from build123d import *

# Parameters (mm, degrees)
BOSS_EXTRUDE1_DEPTH = 40
BOSS_EXTRUDE2_DEPTH = 7
BOSS_EXTRUDE3_START = 25
BOSS_EXTRUDE3_DEPTH = 25
BOSS_EXTRUDE4_START = -12
BOSS_EXTRUDE4_DEPTH = 3


with BuildPart() as part:
    # Sketch1 → Boss-Extrude1 (new body)
    with BuildSketch(Plane.XY):
        with BuildLine():
            Line((-2.25, 5.25), (2.25, 5.25))
            ThreePointArc((2.25, 5.25), (4.371320344, 4.371320344), (5.25, 2.25))
            Line((5.25, 2.25), (5.25, -2.25))
            ThreePointArc((5.25, -2.25), (4.371320344, -4.371320344), (2.25, -5.25))
            Line((2.25, -5.25), (-2.25, -5.25))
            ThreePointArc((-2.25, -5.25), (-4.371320344, -4.371320344), (-5.25, -2.25))
            Line((-5.25, -2.25), (-5.25, 2.25))
            ThreePointArc((-5.25, 2.25), (-4.371320344, 4.371320344), (-2.25, 5.25))
        make_face()
    extrude(amount=BOSS_EXTRUDE1_DEPTH)

    # Sketch2 → Boss-Extrude2 (add)
    with BuildSketch(Plane.XY):
        with BuildLine():
            Line((8.999999945, -3.000810302), (8.999999945, 2.999189698))
            ThreePointArc((8.999999945, 2.999189698), (8.121463527, 5.120366794), (6.000405096, 5.999189671))
            Line((6.000405096, 5.999189671), (-5.999594794, 6.000810275))
            ThreePointArc((-5.999594794, 6.000810275), (-8.121177041, 5.122273883), (-8.999999945, 3.000810302))
            Line((-8.999999945, 3.000810302), (-8.999999945, -2.999189698))
            ThreePointArc((-8.999999945, -2.999189698), (-8.121463527, -5.120366794), (-6.000405096, -5.999189671))
            Line((-6.000405096, -5.999189671), (5.999594794, -6.000810275))
            ThreePointArc((5.999594794, -6.000810275), (8.121177041, -5.122273883), (8.999999945, -3.000810302))
        make_face()
    extrude(amount=-BOSS_EXTRUDE2_DEPTH)

    # Sketch3 → Boss-Extrude3 (add)
    with BuildSketch(Plane.XY.offset(BOSS_EXTRUDE3_START)):
        with BuildLine():
            Line((0.000405151, 5.25), (-5.999999945, 5.25))
            ThreePointArc((-5.999999945, 5.25), (-7.590417233, 4.59122759), (-8.249189643, 3.000810302))
            Line((-8.249189643, 3.000810302), (-8.249189643, -2.999189698))
            ThreePointArc((-8.249189643, -2.999189698), (-7.590631979, -4.58939221), (-6.000607381, -5.248379314))
            Line((-6.000607381, -5.248379314), (0.000405151, -5.25))
            Line((0.000405151, -5.25), (0.000405151, -6.000000082))
            Line((0.000405151, -6.000000082), (-6.000405096, -5.999189671))
            ThreePointArc((-6.000405096, -5.999189671), (-8.121463527, -5.120366794), (-8.999999945, -2.999189698))
            Line((-8.999999945, -2.999189698), (-8.999999945, 3.000810302))
            ThreePointArc((-8.999999945, 3.000810302), (-8.121177041, 5.122273883), (-5.999594794, 6.000810275))
            Line((-5.999594794, 6.000810275), (0.000405151, 5.999999973))
            Line((0.000405151, 5.999999973), (0.000405151, 5.25))
        make_face()
    extrude(amount=-BOSS_EXTRUDE3_DEPTH)

    # Sketch5 → Boss-Extrude4 (add)
    with BuildSketch(Plane.XY.offset(40).offset(BOSS_EXTRUDE4_START)):
        with BuildLine():
            Line((0.000405151, -6.000000082), (5.999594794, -6.000810275))
            ThreePointArc((5.999594794, -6.000810275), (8.121177041, -5.122273883), (8.999999945, -3.000810302))
            Line((8.999999945, -3.000810302), (8.999999945, 2.999189698))
            ThreePointArc((8.999999945, 2.999189698), (8.121463527, 5.120366794), (6.000405096, 5.999189671))
            Line((6.000405096, 5.999189671), (0.000405151, 5.999999973))
            Line((0.000405151, 5.999999973), (-5.999594794, 6.000810275))
            ThreePointArc((-5.999594794, 6.000810275), (-8.121177041, 5.122273883), (-8.999999945, 3.000810302))
            Line((-8.999999945, 3.000810302), (-8.999999945, -2.999189698))
            ThreePointArc((-8.999999945, -2.999189698), (-8.121463527, -5.120366794), (-6.000405096, -5.999189671))
            Line((-6.000405096, -5.999189671), (0.000405151, -6.000000082))
        make_face()
    extrude(amount=-BOSS_EXTRUDE4_DEPTH)


solid = part.part
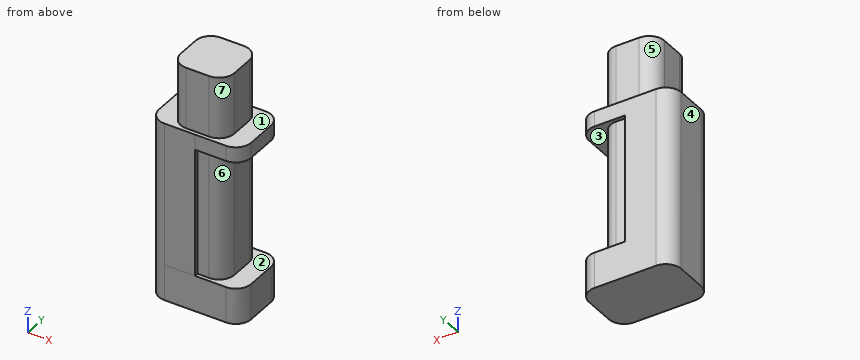
For this review, take the finished solid that the model builds, in its own axes (mm). Face numbers are marked on the shaded views. A direction names the side the tool comes from. Give positions to 0.01 mm unless a question says otherwise; leave off trailing zeros. Order: outer loops, then holes, each group sorted by start corner. A loop starts at its lowest first (then second) coordinate and runs counter-clockwise, first axis right, second up. Notation, with made-up numbers: M 80.25,85.5 L 102.25,85.5 A22 cw 102.25,112.5 Z; hole C 16,74.5 d9. An arc over 180 degrees is marked long. Answer in a Markdown table with one row per item. Add a question column.
(1) Mouldability with a two-part tool opening along Z and no side actions: class the marked faces 1, 2, 3 and 4 as +Z half, -Z half, draft (parallel to the pull), parting line (faces both ways), or undercut.
(2) Consider section D-D on z = -2.5. State the section outline as (x, y) points, and give its area (3 significant figures).
(3) Consider section A-A on z = 6. State the section outline as (x, y) points, and give its area (3 significant figures).
(4) Consider section B-B on y = 0.75. State the section outline as (x, z) points, and give its area (3 significant figures).
(5) Consider section C-C on x = 6.75. State the section outline as (y, z) points.
(6) Wall thickness on probe 1 along Z at (x, y) = (7.5, -0.75); probe 2 along X at (y, z) = (1.25, 23); probe 3 along Y at (x, z) = (2.5, 32.5): over which ranges is each line inside the solid? List them lowest first. Write a range as [from, to].
(7) For the marked faces 5, 6 and 7, list the 3-axis set-ups (+Z, -Z, +X, -X, +Y, -Y) from which the entire face can be reached by the end or side of a thin tool; tool diameter is ignored.
(8) For pin 1 (1.3 mm diameter, centred on y = 1, z = 35, fed in from +X); pin 2 (0.6 mm diameter, centred on y = -6, z = 8, fed in from +X); pin 3 (5 mm diameter, centred on x = 0.5, z = 33.5, fed in from -Y), all flat-tipped, find the tip position at first contact; note any pin that passes through.
Evaluation:
| question | item | result |
|---|---|---|
| 1 | face 1 | +Z half |
| 1 | face 2 | undercut |
| 1 | face 3 | undercut |
| 1 | face 4 | draft |
| 2 | outline | M -9,-3 A3 ccw -6,-6 L 6,-6 A3 ccw 9,-3 L 9,3 A3 ccw 6,6 L -6,6 A3 ccw -9,3 Z |
| 2 | area | 208 mm^2 |
| 3 | outline | M -9,-3 A3 ccw -6,-6 L 0,-6 L 0,-5.25 L 2.25,-5.25 A3 ccw 5.25,-2.25 L 5.25,2.25 A3 ccw 2.25,5.25 L 0,5.25 L 0,6 L -6,6 A3 ccw -9,3 Z; hole M -8.25,-3 A2.25 ccw -6,-5.25 L -2.31,-5.25 A3 cw -5.25,-2.25 L -5.25,2.25 A3 cw -2.25,5.25 L -6,5.25 A2.25 ccw -8.25,3 Z |
| 3 | area | 122 mm^2 |
| 4 | outline | M -9,-7 L 9,-7 L 9,0 L 5.25,0 L 5.25,25 L 9,25 L 9,28 L 5.25,28 L 5.25,40 L -5.25,40 L -5.25,28 L -9,28 Z; hole M -8.25,0 L -5.25,0 L -5.25,25 L -8.25,25 Z |
| 4 | area | 587 mm^2 |
| 5 | outline | M -5.91,-7 L 5.9,-7 L 5.9,0 L -5.91,0 Z; M -5.91,25 L 5.9,25 L 5.9,28 L -5.91,28 Z |
| 6 | probe 1 | z = [-7, 0], [25, 28] |
| 6 | probe 2 | x = [-9, -8.25], [-5.25, 5.25] |
| 6 | probe 3 | y = [-5.24, 5.24] |
| 7 | face 5 | +Z, -X, +Y |
| 7 | face 6 | +X, -Y |
| 7 | face 7 | +Z, +X, -Y |
| 8 | pin 1 | stops at x = 5.25 |
| 8 | pin 2 | stops at x = 0 |
| 8 | pin 3 | stops at y = -5.25 |
